from build123d import *

# Parameters (mm, degrees)
PAD004_DEPTH        = 3
FILLET009_R         = 2
HOLE002_D           = 2.2
HOLE002_DEPTH       = 20
HOLE002_CSINK_D     = 4.4
HOLE002_CSINK_ANGLE = 90


with BuildPart() as part:
    # Sketch016 → Pad004 (new body)
    with BuildSketch(Plane.XY.offset(-1.4)):
        Polygon((120, 48.4), (120, 8.4), (-120, 8.4), (-120, 48.4), (-15, 48.4), (-15, 18.4), (15, 18.4), (15, 48.4), align=None)
    extrude(amount=PAD004_DEPTH)

    # Fillet009
    fillet009_edges = [part.edges().sort_by_distance(p)[0] for p in [
        (-120, 48.4, 0.1),
        (-120, 8.4, 0.1),
        (120, 8.4, 0.1),
        (120, 48.4, 0.1),
        (15, 48.4, 0.1),
        (-15, 48.4, 0.1),
        (-15, 18.4, 0.1),
        (15, 18.4, 0.1),
    ]]
    fillet(fillet009_edges, radius=FILLET009_R)

    # Hole002
    with Locations(Plane.XY.offset(1.6)):
        with Locations((-110, 28.4), (110, 28.4)):
            CounterSinkHole(HOLE002_D / 2, HOLE002_CSINK_D / 2, depth=HOLE002_DEPTH, counter_sink_angle=HOLE002_CSINK_ANGLE)


solid = part.part
Geometry: final body of the model. Coordinates: model frame, mm. Give positions to 0.01 mm unless a question says otherwise; leave off trailing zeros. Write each loop counter-clockwise with the first axis right and the second up, starting at its lowest first coordinate (ties: lowest second). Pieces come first, ordered by that corner, then holes. Notation, with made-up numbers: (63.5, 5) -> (87.5, 5) arc R18 ccw to (87.5, 22) -> close; hole circle Ø7 at (31.25, 37.5). An arc over 180 degrees is marked (long way). Answer in a Markdown table with one row per item.
(1) Section query A-A on z = -0.45. Return loops of the section in (x, y), then the cut area to 3 significant figures.
Answers below:
| item | result |
|---|---|
| outline | (-120, 10.4) arc R2 ccw to (-118, 8.4) -> (118, 8.4) arc R2 ccw to (120, 10.4) -> (120, 46.4) arc R2 ccw to (118, 48.4) -> (17, 48.4) arc R2 ccw to (15, 46.4) -> (15, 20.4) arc R2 cw to (13, 18.4) -> (-13, 18.4) arc R2 cw to (-15, 20.4) -> (-15, 46.4) arc R2 ccw to (-17, 48.4) -> (-118, 48.4) arc R2 ccw to (-120, 46.4) -> close; hole circle Ø2.2 at (-110, 28.4); hole circle Ø2.2 at (110, 28.4) |
| area | 8,690 mm^2 |
(2) Draft query along Y for faces 1 (the flat face through (2, 15, -1.4)), 2 (the conical face through (110, 30, 1)). Return one class per face: +Y half, -Y half, draft (parallel to the pull), parting line (faces both ways), or undercut.
Answers below:
| item | result |
|---|---|
| face 1 | draft |
| face 2 | undercut |
(3) Ray query, line 1 along X through (y, z) = (28.4, -0.8); line 2 along Y through (x, z) = (-110, -0.9); line 3 along X through (y, z) = (45, 1). Return the intervals inside material, ascending. Write a range as [from, to].
Answers below:
| item | result |
|---|---|
| line 1 | [-120, -111.1], [-108.9, -15], [15, 108.9], [111.1, 120] |
| line 2 | [8.4, 27.3], [29.5, 48.4] |
| line 3 | [-120, -15], [15, 120] |
(4) Section query B-B on y = 35. Return loops of the section in (x, z), then the cut area to 3 significant figures.
Answers below:
| item | result |
|---|---|
| outline | (-120, -1.4) -> (-15, -1.4) -> (-15, 1.6) -> (-120, 1.6) -> close; (15, -1.4) -> (120, -1.4) -> (120, 1.6) -> (15, 1.6) -> close |
| area | 630 mm^2 |
(5) Pin query (flat end, axial travel): pin 1 (2 mm diameter, centred on x = 110, y = 28.4, fed in from -Z); pin 2 (0.9 mm diameter, centred on x = -5.5, z = -0.5, fed in from +Y). Return the tip coordinate at first contact, or that it passes through.
Answers below:
| item | result |
|---|---|
| pin 1 | through |
| pin 2 | y = 18.4 |
(6) Section query C-C on x = -3.5. Return loops of the section in (y, z), then the cut area to 3 significant figures.
Answers below:
| item | result |
|---|---|
| outline | (8.4, -1.4) -> (18.4, -1.4) -> (18.4, 1.6) -> (8.4, 1.6) -> close |
| area | 30.0 mm^2 |
